For this review, take the finished solid that the model builds, in its own axes (mm). A direction names the side the tool comes from. Coordinates: 2 decimals unless noted, no trailing zeros. Loops run counter-clockwise (first coordinate to the right, second up) from the corner with the lowest first, then second, coordinate; pieces in that order, holes last. Notation, with made-up numbers: M 62,-28 L 108,-28 A12 ccw 108,-19 Z; hole C 46.5,39 d11. An arc over 180 degrees is marked long. Use one line per item in the form item = value.
```python
from build123d import *

# Parameters (mm, degrees)
SKETCH1_R               = 9.5
SKETCH1_R_2             = 8.5
BOSS_EXTRUDE1_DEPTH     = 12
SKETCH2_R               = 13.4
SKETCH2_R_2             = 8.5
BOSS_EXTRUDE2_DEPTH     = 10
SKETCH3_W               = 2
SKETCH3_H               = 22
CUT_EXTRUDE1_DEPTH      = 21
BOSS_EXTRUDE3_DEPTH     = 10
SKETCH4_R               = 1.6
CUT_EXTRUDE2_DEPTH      = 21
CUT_EXTRUDE2_DEPTH_BACK = 21
CHAMFER1_SIZE           = 1


with BuildPart() as part:
    # Sketch1 → Boss-Extrude1 (new body)
    with BuildSketch(Plane(origin=(0, 0, 0), x_dir=(1, 0, 0), z_dir=(0, 1, 0))):
        Circle(SKETCH1_R)
        Circle(SKETCH1_R_2, mode=Mode.SUBTRACT)
    extrude(amount=BOSS_EXTRUDE1_DEPTH)

    # Sketch2 → Boss-Extrude2 (add)
    with BuildSketch(Plane(origin=(0, 12, 0), x_dir=(1, 0, 0), z_dir=(0, 1, 0))):
        Circle(SKETCH2_R)
        Circle(SKETCH2_R_2, mode=Mode.SUBTRACT)
    extrude(amount=BOSS_EXTRUDE2_DEPTH)

    # Sketch3 → Cut-Extrude1 (cut)
    with BuildSketch(Plane(origin=(0, 0, 0), x_dir=(0, 0, -1), z_dir=(1, 0, 0))):
        with Locations((0, 11)):
            Rectangle(SKETCH3_W, SKETCH3_H)
    extrude(amount=-CUT_EXTRUDE1_DEPTH, mode=Mode.SUBTRACT)

    # Sketch6 → Boss-Extrude3 (add)
    with BuildSketch(Plane(origin=(0, 22, 0), x_dir=(1, 0, 0), z_dir=(0, 1, 0))):
        Polygon((-9.518301515, -1), (-14.563720806, -1), (-14.563720806, -11.949530953), (-6.063720806, -11.949530953), align=None)
        Polygon((-6.063720806, 11.949530953), (-14.563720806, 11.949530953), (-14.563720806, 1), (-9.518301515, 1), align=None)
    extrude(amount=-BOSS_EXTRUDE3_DEPTH)

    # Sketch4 → Cut-Extrude2 (cut, two sides)
    with BuildSketch(Plane.XY.offset(-1)) as cut_extrude2_sk:
        with Locations((-10.901802989, 17)):
            Circle(SKETCH4_R)
    extrude(amount=CUT_EXTRUDE2_DEPTH, mode=Mode.SUBTRACT)
    extrude(cut_extrude2_sk.sketch, amount=-CUT_EXTRUDE2_DEPTH_BACK, mode=Mode.SUBTRACT)

    # Chamfer1
    chamfer1_edges = [part.edges().sort_by_distance(p)[0] for p in [
        (0.500870333, 22, -8.485230045),
        (-11.502346157, 22, 1),
        (-11.502346157, 22, -1),
        (13.4, 22, 0),
        (13.4, 12, 0),
        (-10.313720806, 22, 11.949530953),
        (-14.563720806, 22, 6.474765476),
        (-10.313720806, 12, 11.949530953),
        (-14.563720806, 12, 6.474765476),
        (-10.313720806, 22, -11.949530953),
        (-14.563720806, 22, -6.474765476),
        (-14.563720806, 12, -6.474765476),
        (-10.313720806, 12, -11.949530953),
    ]]
    chamfer(chamfer1_edges, length=CHAMFER1_SIZE)


solid = part.part
```
1. For pin 1 Ø2 at (y, z) = (18.5, 5.5) entering from +X; pin 2 Ø6.5 at (x, y) = (-11, 14.5) entering from -Z; pin 3 Ø1.8 at (x, y) = (-11, 14.5) entering from +Z; pin 4 Ø8 at (x, z) = (8, 3.5) entering from -Y, all flat-tipped, find the tip position at first contact; note any pin that passes through.
Computed values:
pin_1 = 12.62
pin_2 = -11.95
pin_3 = 11.95
pin_4 = 0
2. Consider section C-C on z = 4.25. State how many separate pieces and enclosed holes the cut face has, plus the area to 3 significant figures.
Computed values:
separate_pieces = 2
enclosed_holes = 1
area = 141 mm2
3. Consider section D-D on y = 10.75. Write out the cut boundary in (x, z), plus the area to 3 significant figures.
Computed values:
outline = M -9.45,-1 A9.5 ccw long -9.45,1 L -8.44,1 A8.5 cw long -8.44,-1 Z
area = 54.5 mm2
4. Wall thickness on line 1 along X through (y, z) = (17, 7); line 2 along X through (y, z) = (17, 5.25); line 3 along Z through (x, y) = (-8.5, 20.5): over which ranges is each line inside the solid? List them lowest first. Write a range as from..to.
Computed values:
line_1 = -14.56..-12.5, -9.3..-4.82, 4.82..11.43
line_2 = -14.56..-12.5, -9.3..-6.68, 6.68..12.33
line_3 = -11.95..-1, 1..11.95
5. Consider section B-B on y = 17. Write out the cut boundary in (x, z), plus the area to 3 significant figures.
Computed values:
outline = M -14.56,-11.95 L -12.5,-11.95 L -12.5,-1 L -14.56,-1 Z; M -14.56,1 L -12.5,1 L -12.5,11.95 L -14.56,11.95 Z; M -9.3,-11.95 L -6.06,-11.95 A13.4 ccw long -6.06,11.95 L -9.3,11.95 L -9.3,1 L -8.44,1 A8.5 cw long -8.44,-1 L -9.3,-1 Z
area = 333 mm2
6. Tool access review of faces 5 (the face through (-9.4, 12, 2.6)), 6 (the face through (-9, 16, -11.95)), 7 (the face through (-9, 18, 11.95)), 8 (the face through (-10.13, 21.51, -11.44)), 9 (the face through (-10.13, 12.51, -11.46)): name each direction out of +Z, -Z, +X, -X, +Y, -Y from which nothing blocks a thin tool from reaching the whole face with its end or side.
Computed values:
face_5 = -Y
face_6 = -Z, -X, +Y, -Y
face_7 = +Z, -X, +Y, -Y
face_8 = -Z, -X, +Y
face_9 = -Z, -X, -Y
7. Draft analysis for pull direction Z (two halves, no side actions). For faces 1 (the face through (9.49, 5.92, 0.4)), 2 (the face through (8.65, 21.16, 0.37)), 3 (the face through (-14.564, 17, -7)), 4 (the face through (-11, 13, 1)), state which applies: +Z half, -Z half, draft (parallel to the pull), parting line (faces both ways), or undercut.
Computed values:
face_1 = parting line
face_2 = undercut
face_3 = draft
face_4 = undercut
8. Consider section A-A on x = 0. Write out the cut boundary in (y, z), plus the area to 3 significant figures.
Computed values:
outline = M 0,-9.5 L 12,-9.5 L 12,-12.4 L 13,-13.4 L 21,-13.4 L 22,-12.4 L 22,-9.5 L 21,-8.5 L 0,-8.5 Z; M 0,8.5 L 21,8.5 L 22,9.5 L 22,12.4 L 21,13.4 L 13,13.4 L 12,12.4 L 12,9.5 L 0,9.5 Z
area = 119 mm2
